Check sheet for the modelled part. Datum: model origin and axes. Units: mm. Face numbers are marked on the shaded views. Round coordinates to 2 decimals unless told otherwise and drop trailing zeros. Loops run counter-clockwise (first coordinate to the right, second up) from the corner with the lowest first, then second, coordinate; pieces in that order, holes last. Notation, with made-up numbers: (34, 52) - (56, 52) arc R20 ccw to (56, 84) - close; hole circle Ø8 at (57.5, 60.5). An arc over 180 degrees is marked (long way). Answer in a Markdown table with one row per item. Add a question column.
(1) Gauge pin test, flat ends, axial feed: pin 1 (5 mm diameter, centred on y = -20.5, z = 11.5, fed in from -X); pin 2 (1 mm diameter, centred on x = 1, y = -4.5, fed in from -Z). Record the tip position at first contact, or that the pin passes through.
(2) Cross-section at A-A on x = -0.5. Enter the section's corners in (y, z).
(3) Thickness scan on line 1 along Y through (x, z) = (-4.25, 0); line 2 along Z through (x, y) = (-2.75, -1.5); line 3 along Z through (x, y) = (-3.25, -14). Record the ranges inside material, lowest first.
(4) Mould release check, pull along Y, two halves, no side actions. Record for the marked faces 1 and 2: +Y half, -Y half, draft (parallel to the pull), parting line (faces both ways), or undercut.
from build123d import *

# Parameters (mm, degrees)
FILLET2_R = 0.6
FILLET3_R = 0.5


with BuildPart() as part:
    # Sketch1 → Revolve1 (revolve)
    with BuildSketch(Plane.XY):
        with BuildLine():
            Line((6, 10.200814883), (-6, 10.200814883))
            Line((-6, 10.200814883), (-6, 7.700814883))
            Line((-6, 7.700814883), (-2.645751311, 7.700814883))
            ThreePointArc((-2.645751311, 7.700814883), (0, 8.700814883), (2.645751311, 7.700814883))
            Line((2.645751311, 7.700814883), (6, 7.700814883))
            Line((6, 7.700814883), (6, 10.200814883))
        make_face()
    revolve(axis=Axis((44.126443973, -10.799185117, 0), (-1, 0, 0)))

    # Fillet2
    fillet2_edges = [part.edges().sort_by_distance(p)[0] for p in [
        (-6, -31.799185117, 0),
        (6, -31.799185117, 0),
    ]]
    fillet(fillet2_edges, radius=FILLET2_R)

    # Fillet3
    fillet3_edges = [part.edges().sort_by_distance(p)[0] for p in [
        (-2.645751311, -29.299185117, 0),
        (2.645751311, -29.299185117, 0),
    ]]
    fillet(fillet3_edges, radius=FILLET3_R)


solid = part.part
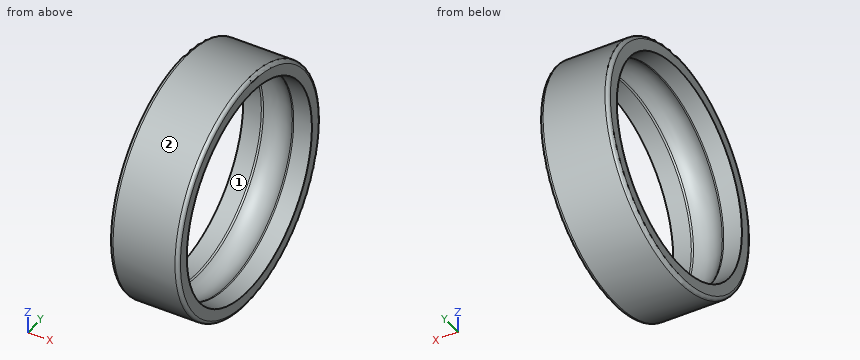
Answers:
| question | item | result |
|---|---|---|
| 1 | pin 1 | passes through |
| 1 | pin 2 | stops at z = -20.18 |
| 2 | outline | circle Ø42 at (-10.8, 0); hole circle Ø38.94 at (-10.8, 0) |
| 3 | line 1 | y = -31.8 to -29.3, 7.7 to 10.2 |
| 3 | line 2 | z = -18.83 to -16, 16 to 18.83 |
| 3 | line 3 | z = -20.75 to -18.22, 18.22 to 20.75 |
| 4 | face 1 | undercut |
| 4 | face 2 | parting line |
